Source: CAD feature listing. Evaluate the final solid. Frame: model axes, mm. Face numbers are marked on the shaded views. A direction names the side the tool comes from. Give positions to 0.01 mm unless a question says otherwise; leave off trailing zeros. Order: outer loops, then holes, each group sorted by start corner. A loop starts at its lowest first (then second) coordinate and runs counter-clockwise, first axis right, second up. Notation, with made-up numbers: M -17,-6 L 21,-6 A33 cw 21,30 Z; hole C 60,-32.5 d3. An arc over 180 degrees is marked long. Answer as a JSON object with one key per item and string values. Group by question number.
1. Set-up query: the marked faces 1, 2 and 3. Return all of +Z, -Z, +X, -X, +Y, -Y with unobstructed straight access to the full face (end or side cutting, diameter ignored); none if empty.
2. Material intervals for L1, parallel to Z at x = -13.5, y = 14; L2, parallel to Z at x = 12, y = 7.5; L3, parallel to Z at x = -21.5, y = -20, sorted ascending. Write a range as [from, to].
3. Pull-direction query (Z, two-part tool) for the marked faces 4, 5 and 6; classes: +Z half, -Z half, draft (parallel to the pull), parting line (faces both ways), or undercut.
4. Section query D-D (y = -13). Output: boundary loops of the cut face in (x, z).
5. Section query C-C (x = 0). Output: boundary loops of the cut face in (y, z).
6. Section query B-B (y = 0). Output: boundary loops of the cut face in (x, z), plus the area to 3 significant figures.
7. Pin query (flat end, axial travel): P1, Ø20, axis at y = -7, z = -39.5, coming from the -X side; P2, Ø12, axis at y = -7.5, z = -34.5, coming from the +X side; P3, Ø12, axis at x = -16.5, z = -17, coming from the -Y side; P4, Ø1, axis at x = -16.5, z = -52.5, coming from the +Y side. Return the tip coordinate at first contact, or that it passes through.
8. Section query A-A (x = 16.5). Output: boundary loops of the cut face in (y, z), plus the area to 3 significant figures.
from build123d import *

# Parameters (mm, degrees)
SKETCH1_R           = 15
BOSS_EXTRUDE1_DEPTH = 15
SKETCH2_R           = 20
BOSS_EXTRUDE2_DEPTH = 6
SKETCH3_R           = 11
BOSS_EXTRUDE3_DEPTH = 15
BOSS_EXTRUDE4_START = 5
SKETCH4_W           = 29.8
SKETCH4_H           = 40
BOSS_EXTRUDE4_DEPTH = 61.5
SKETCH5_R           = 30
BOSS_EXTRUDE5_DEPTH = 1


with BuildPart() as part:
    # Sketch1 → Boss-Extrude1 (new body)
    with BuildSketch(Plane.XY):
        Circle(SKETCH1_R)
    extrude(amount=BOSS_EXTRUDE1_DEPTH)

    # Sketch2 → Boss-Extrude2 (add)
    with BuildSketch(Plane.XY.offset(15)):
        Circle(SKETCH2_R)
    extrude(amount=BOSS_EXTRUDE2_DEPTH)

    # Sketch3 → Boss-Extrude3 (add)
    with BuildSketch(Plane(origin=(0, 0, 0), x_dir=(-1, 0, 0), z_dir=(0, 0, -1))):
        with Locations(Location((0, 0, 0), (0, 0, 180))):
            Circle(SKETCH3_R)
    extrude(amount=BOSS_EXTRUDE3_DEPTH)

    # Sketch4 → Boss-Extrude4 (add)
    with BuildSketch(Plane(origin=(0, 0, 0), x_dir=(-1, 0, 0), z_dir=(0, 0, -1)).offset(BOSS_EXTRUDE4_START)):
        Rectangle(SKETCH4_W, SKETCH4_H)
    extrude(amount=BOSS_EXTRUDE4_DEPTH)

    # Sketch5 → Boss-Extrude5 (add)
    with BuildSketch(Plane(origin=(0, 0, 0), x_dir=(-1, 0, 0), z_dir=(0, 0, -1))):
        Circle(SKETCH5_R)
    extrude(amount=-BOSS_EXTRUDE5_DEPTH)


solid = part.part
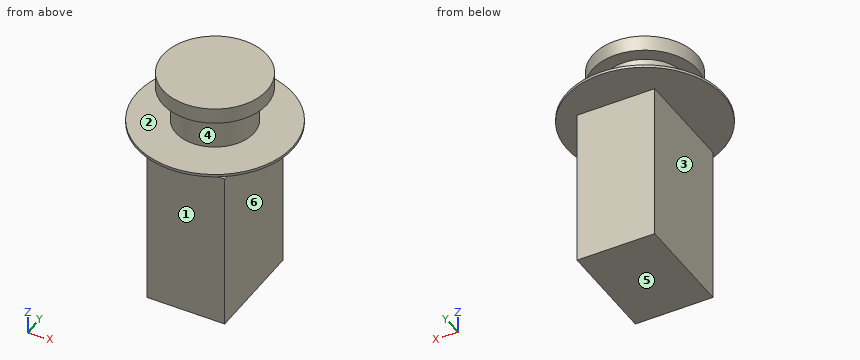
Answer sheet:
{
 "1": {"face 1": "-Z, +X, -X, -Y", "face 2": "none", "face 3": "-Z, -X, +Y, -Y"},
 "2": {"L1": "[-66.5, -5], [0, 1], [15, 21]", "L2": "[-66.5, -5], [0, 21]", "L3": "[0, 1]"},
 "3": {"face 4": "undercut", "face 5": "-Z half", "face 6": "draft"},
 "4": {"outline": "M -27.04,0 L 27.04,0 L 27.04,1 L 7.48,1 L 7.48,15 L 15.2,15 L 15.2,21 L -15.2,21 L -15.2,15 L -7.48,15 L -7.48,1 L -27.04,1 Z; M -14.9,-66.5 L 14.9,-66.5 L 14.9,-5 L -14.9,-5 Z"},
 "5": {"outline": "M -30,0 L -11,0 L -11,-5 L -20,-5 L -20,-66.5 L 20,-66.5 L 20,-5 L 11,-5 L 11,0 L 30,0 L 30,1 L 15,1 L 15,15 L 20,15 L 20,21 L -20,21 L -20,15 L -15,15 L -15,1 L -30,1 Z"},
 "6": {"outline": "M -30,0 L -11,0 L -11,-5 L -14.9,-5 L -14.9,-66.5 L 14.9,-66.5 L 14.9,-5 L 11,-5 L 11,0 L 30,0 L 30,1 L 15,1 L 15,15 L 20,15 L 20,21 L -20,21 L -20,15 L -15,15 L -15,1 L -30,1 Z", "area": "2,660 mm^2"},
 "7": {"P1": "x = -14.9", "P2": "x = 14.9", "P3": "y = -20", "P4": "through"},
 "8": {"outline": "M -25.05,0 L 25.05,0 L 25.05,1 L -25.05,1 Z; M -11.3,15 L 11.3,15 L 11.3,21 L -11.3,21 Z", "area": "186 mm^2"}
}
